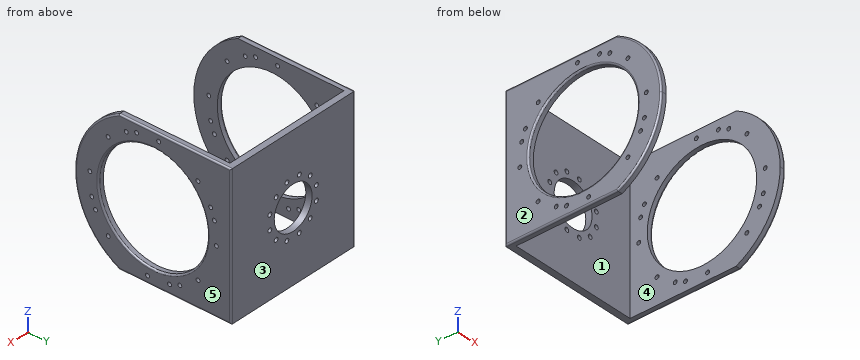
```python
from build123d import *

# Parameters (mm, degrees)
EXTRUDE_1_DEPTH          = 180
SKETCH_2_R               = 27.5
CUT_EXTRUDE_1_DEPTH      = 180
SKETCH_3_R               = 70
CUT_EXTRUDE_2_DEPTH      = 217
CUT_EXTRUDE_5_DEPTH      = 324.728281125
CUT_EXTRUDE_5_DEPTH_BACK = 324.728281125
FILLET_2_R               = 2
CUT_EXTRUDE_6_DEPTH      = 324.728281298
CUT_EXTRUDE_6_DEPTH_BACK = 324.728281298
SKETCH_10_R              = 2.5
SKETCH_11_R              = 2.75
CUT_EXTRUDE_7_DEPTH      = 29


with BuildPart() as part:
    # 草图1 → 凸台-拉伸1 (new body)
    with BuildSketch(Plane.XY):
        Polygon((-90, 200), (90, 200), (90, 0), (82.8, 0), (82.8, 192), (-82.8, 192), (-82.8, 0), (-90, 0), align=None)
    extrude(amount=EXTRUDE_1_DEPTH)

    # 草图2 → 切除-拉伸1 (cut)
    with BuildSketch(Plane(origin=(0, 200, 0), x_dir=(1, 0, 0), z_dir=(0, 1, 0))):
        with Locations(Location((0, -90, 0), (0, 0, 270))):
            Circle(SKETCH_2_R)
    extrude(amount=-CUT_EXTRUDE_1_DEPTH, mode=Mode.SUBTRACT)

    # 草图3 → 切除-拉伸2 (cut)
    with BuildSketch(Plane(origin=(90, 0, 0), x_dir=(0, 0, -1), z_dir=(1, 0, 0))):
        with Locations(Location((-90, 100, 0), (0, 0, 90))):
            Circle(SKETCH_3_R)
    extrude(amount=-CUT_EXTRUDE_2_DEPTH, mode=Mode.SUBTRACT)

    # 草图9 → 切除-拉伸5 (cut, two sides: drawn at the far end of the back side and taken through both)
    with BuildSketch(Plane(origin=(90, 0, 0), x_dir=(0, 0, -1), z_dir=(1, 0, 0)).offset(-CUT_EXTRUDE_5_DEPTH_BACK)):
        with BuildLine():
            Line((0, 0), (0, 56.411010565))
            ThreePointArc((0, 56.411010565), (-36.891144692, 15.268367844), (-90.000000357, 0))
            Line((-90.000000357, 0), (0, 0))
        make_face()
        with BuildLine():
            Line((-180, 0), (-90.000000357, 0))
            ThreePointArc((-90.000000357, 0), (-143.108855611, 15.268368034), (-180, 56.411010565))
            Line((-180, 56.411010565), (-180, 0))
        make_face()
    extrude(amount=CUT_EXTRUDE_5_DEPTH + CUT_EXTRUDE_5_DEPTH_BACK, mode=Mode.SUBTRACT)

    # 圆角2
    fillet_2_edges = [part.edges().sort_by_distance(p)[0] for p in [
        (-90, 128.205505282, 0),
        (-90, 128.205505282, 180),
        (-90, 200, 90),
        (90, 200, 90),
        (-90, 30, 90),
        (90, 30, 90),
        (90, 128.205505282, 0),
        (90, 0, 90),
        (-90, 0, 90),
        (90, 128.205505282, 180),
    ]]
    fillet(fillet_2_edges, radius=FILLET_2_R)

    # 草图10 → 切除-拉伸6 (cut, two sides: drawn at the far end of the back side and taken through both)
    with BuildSketch(Plane(origin=(90, 0, 0), x_dir=(0, 0, -1), z_dir=(1, 0, 0)).offset(-CUT_EXTRUDE_6_DEPTH_BACK)):
        with Locations(Location((-32.609998318, 157.514782508, 0), (0, 0, 90))):
            Circle(SKETCH_10_R)
        with Locations(Location((-16.325246691, 134.257746931, 0), (0, 0, 90))):
            Circle(SKETCH_10_R)
        with Locations(Location((-11.541409366, 121.114261903, 0), (0, 0, 90))):
            Circle(SKETCH_10_R)
        with Locations(Location((-9.066918551, 92.830702464, 0), (0, 0, 90))):
            Circle(SKETCH_10_R)
        with Locations(Location((-32.485217492, 42.609998318, 0), (0, 0, 90))):
            Circle(SKETCH_10_R)
        with Locations(Location((-55.742253069, 26.325246691, 0), (0, 0, 90))):
            Circle(SKETCH_10_R)
        with Locations(Location((-68.885738097, 21.541409366, 0), (0, 0, 90))):
            Circle(SKETCH_10_R)
        with Locations(Location((-97.169297536, 19.066918551, 0), (0, 0, 90))):
            Circle(SKETCH_10_R)
        with Locations(Location((-147.390001682, 42.485217492, 0), (0, 0, 90))):
            Circle(SKETCH_10_R)
        with Locations(Location((-163.674753309, 65.742253069, 0), (0, 0, 90))):
            Circle(SKETCH_10_R)
        with Locations(Location((-168.458590634, 78.885738097, 0), (0, 0, 90))):
            Circle(SKETCH_10_R)
        with Locations(Location((-170.933081449, 107.169297536, 0), (0, 0, 90))):
            Circle(SKETCH_10_R)
        with Locations(Location((-147.514782508, 157.390001682, 0), (0, 0, 90))):
            Circle(SKETCH_10_R)
        with Locations(Location((-124.257746931, 173.674753309, 0), (0, 0, 90))):
            Circle(SKETCH_10_R)
        with Locations(Location((-111.114261903, 178.458590634, 0), (0, 0, 90))):
            Circle(SKETCH_10_R)
        with Locations(Location((-82.830702464, 180.933081449, 0), (0, 0, 90))):
            Circle(SKETCH_10_R)
    extrude(amount=CUT_EXTRUDE_6_DEPTH + CUT_EXTRUDE_6_DEPTH_BACK, mode=Mode.SUBTRACT)

    # 草图11 → 切除-拉伸7 (cut)
    with BuildSketch(Plane.XZ.offset(-192)):
        with Locations(Location((9.058666579, 123.80740392, 0), (0, 0, 270))):
            Circle(SKETCH_11_R)
        with Locations(Location((24.748737342, 114.748737342, 0), (0, 0, 270))):
            Circle(SKETCH_11_R)
        with Locations(Location((33.80740392, 99.058666579, 0), (0, 0, 270))):
            Circle(SKETCH_11_R)
        with Locations(Location((33.80740392, 80.941333421, 0), (0, 0, 270))):
            Circle(SKETCH_11_R)
        with Locations(Location((24.748737342, 65.251262658, 0), (0, 0, 270))):
            Circle(SKETCH_11_R)
        with Locations(Location((9.058666579, 56.19259608, 0), (0, 0, 270))):
            Circle(SKETCH_11_R)
        with Locations(Location((-9.058666579, 56.19259608, 0), (0, 0, 270))):
            Circle(SKETCH_11_R)
        with Locations(Location((-24.748737342, 65.251262658, 0), (0, 0, 270))):
            Circle(SKETCH_11_R)
        with Locations(Location((-33.80740392, 80.941333421, 0), (0, 0, 270))):
            Circle(SKETCH_11_R)
        with Locations(Location((-33.80740392, 99.058666579, 0), (0, 0, 270))):
            Circle(SKETCH_11_R)
        with Locations(Location((-24.748737342, 114.748737342, 0), (0, 0, 270))):
            Circle(SKETCH_11_R)
        with Locations(Location((-9.058666579, 123.80740392, 0), (0, 0, 270))):
            Circle(SKETCH_11_R)
    extrude(amount=-CUT_EXTRUDE_7_DEPTH, mode=Mode.SUBTRACT)


solid = part.part
```
Build history of the part. All positions in model axes, mm. Face numbers are marked on the shaded views. A direction names the side the tool comes from. Round coordinates to 2 decimals unless told otherwise and drop trailing zeros. Write each loop counter-clockwise with the first axis right and the second up, starting at its lowest first coordinate (ties: lowest second). Pieces come first, ordered by that corner, then holes. Notation, with made-up numbers: (72, 15) - (128, 15) arc R21 cw to (128, 27) - close; hole circle Ø10 at (-8.75, -35.75). An arc over 180 degrees is marked (long way). Answer as CSV lines item,"result".
Q1. Cut at C-C (x = -47.5). Write the cut outline in (y, z), and give its area (3 significant figures).
Report:
outline,"(192, 0) - (200, 0) - (200, 180) - (192, 180) - close"
area,"1,440 mm^2"
Q2. Cut at A-A (y = 100). Write the cut outline in (x, z).
Report:
outline,"(-90, 2) arc R2 ccw to (-88, 0) - (-82.8, 0) - (-82.8, 20) - (-88, 20) arc R2 ccw to (-90, 18) - close; (-90, 162) arc R2 ccw to (-88, 160) - (-82.8, 160) - (-82.8, 180) - (-88, 180) arc R2 ccw to (-90, 178) - close; (82.8, 0) - (88, 0) arc R2 ccw to (90, 2) - (90, 18) arc R2 ccw to (88, 20) - (82.8, 20) - close; (82.8, 160) - (88, 160) arc R2 ccw to (90, 162) - (90, 178) arc R2 ccw to (88, 180) - (82.8, 180) - close"
Q3. Pull direction X, two halves, no side cores. Call the marked faces 1, 2 and 3: +X half, -X half, draft (parallel to the pull), parting line (faces both ways), or undercut.
Report:
face 1,"undercut"
face 2,"-X half"
face 3,"draft"
Q4. Tool access for the marked faces 4 and 5: list every direction of +Z, -Z, +X, -X, +Y, -Y with a clear straight run to the whole face (end or side of a thin tool).
Report:
face 4,"+Z, -Z, -Y"
face 5,"+Z, -Z, +X, +Y, -Y"
Q5. Drill centre lines: probe 1 along X at (y, z) = (194, 90); probe 2 along X at (y, z) = (156, 11); probe 3 along Y at (x, z) = (29, 158.5). Where is each one in solid material? Low to high. Write a range as [from, to].
Report:
probe 1,"x = [-90, -27.5], [27.5, 90]"
probe 2,"x = [-90, -82.8], [82.8, 90]"
probe 3,"y = [192, 200]"
Q6. Drop flat-ended pins along their axis: pin 1 (12 mm diameter, centred on y = 29, z = 20, fed in from -X); pin 2 (4.5 mm diameter, centred on y = 121.11, z = 11.54, fed in from +X); pin 3 (7 mm diameter, centred on x = -9.06, z = 56.19, fed in from -Y); pin 4 (5 mm diameter, centred on y = 162, z = 120.5, fed in from +X). Give the stop position or say it passes through.
Report:
pin 1,"stops at x = -90"
pin 2,"passes through"
pin 3,"stops at y = 192"
pin 4,"stops at x = 89.96"
Q7. Cut at B-B (x = 0). Write the cut outline in (y, z), and give its area (3 significant figures).
Report:
outline,"(192, 0) - (200, 0) - (200, 62.5) - (192, 62.5) - close; (192, 117.5) - (200, 117.5) - (200, 180) - (192, 180) - close"
area,"1,000 mm^2"
